from build123d import *

# Parameters (mm, degrees)
SKETCH_1_W          = 49
SKETCH_1_H          = 63
EXTRUDE_1_DEPTH     = 4
SKETCH_2_W          = 45
SKETCH_2_H          = 4
SKETCH_2_W_2        = 4
SKETCH_2_H_2        = 59
EXTRUDE_2_DEPTH     = 26
SKETCH_3_W          = 14
SKETCH_3_H          = 8
SKETCH_3_W_2        = 30
EXTRUDE_3_DEPTH     = 7.2
SKETCH_5_R          = 5.3
CUT_EXTRUDE_1_DEPTH = 4
SKETCH_7_W          = 1.7
SKETCH_7_H          = 1.7
CUT_EXTRUDE_3_DEPTH = 6
SKETCH_8_W          = 1.7
SKETCH_8_H          = 1.7
CUT_EXTRUDE_4_DEPTH = 6
SKETCH_9_W          = 1.7
SKETCH_9_H          = 1.7
CUT_EXTRUDE_5_DEPTH = 6
FILLET_1_R          = 1
SKETCH_6_W          = 1.7
SKETCH_6_H          = 1.7
CUT_EXTRUDE_7_DEPTH = 5
SKETCH_10_W         = 15
SKETCH_10_H         = 27.7
EXTRUDE_4_DEPTH     = 2
CUT_EXTRUDE_8_DEPTH = 13
SKETCH_12_W         = 1.7
SKETCH_12_H         = 1.7
CUT_EXTRUDE_9_DEPTH = 5


with BuildPart() as part:
    # Эскиз1 → Бобышка-Вытянуть1 (new body)
    with BuildSketch(Plane.XY):
        with Locations((2.204545455, -4.295454545)):
            Rectangle(SKETCH_1_W, SKETCH_1_H)
    extrude(amount=EXTRUDE_1_DEPTH)

    # Эскиз2 → Бобышка-Вытянуть2 (add)
    with BuildSketch(Plane(origin=(0, 0, 0), x_dir=(-1, 0, 0), z_dir=(0, 0, -1))):
        with Locations((-0.204545455, 25.204545455)):
            Rectangle(SKETCH_2_W, SKETCH_2_H)
        with Locations((-24.704545455, -6.295454545)):
            Rectangle(SKETCH_2_W_2, SKETCH_2_H_2)
        with Locations((-24.704545455, 25.204545455)):
            Rectangle(SKETCH_2_W_2, SKETCH_2_H)
    extrude(amount=EXTRUDE_2_DEPTH)

    # Эскиз3 → Бобышка-Вытянуть3 (add)
    with BuildSketch(Plane(origin=(0, 0, 0), x_dir=(-1, 0, 0), z_dir=(0, 0, -1))):
        with Locations((-15.704545455, 19.204545455)):
            Rectangle(SKETCH_3_W, SKETCH_3_H)
        with Locations((-7.704545455, -23.795454545)):
            Rectangle(SKETCH_3_W_2, SKETCH_3_H)
    extrude(amount=EXTRUDE_3_DEPTH)

    # Эскиз5 → Вырез-Вытянуть1 (cut)
    with BuildSketch(Plane.ZY.offset(-22.704545455)):
        with Locations((-13, 9.204545455)):
            Circle(SKETCH_5_R)
    extrude(amount=-CUT_EXTRUDE_1_DEPTH, mode=Mode.SUBTRACT)

    # Эскиз7 → Вырез-Вытянуть3 (cut)
    with BuildSketch(Plane.ZY.offset(22.295454545)):
        with Locations((1.75, 24.954545455)):
            Rectangle(SKETCH_7_W, SKETCH_7_H)
    extrude(amount=-CUT_EXTRUDE_3_DEPTH, mode=Mode.SUBTRACT)

    # Эскиз8 → Вырез-Вытянуть4 (cut)
    with BuildSketch(Plane.XZ.offset(35.795454545)):
        with Locations((24.454545455, 1.75)):
            Rectangle(SKETCH_8_W, SKETCH_8_H)
    extrude(amount=-CUT_EXTRUDE_4_DEPTH, mode=Mode.SUBTRACT)

    # Эскиз9 → Вырез-Вытянуть5 (cut)
    with BuildSketch(Plane(origin=(0, 0, -26), x_dir=(-1, 0, 0), z_dir=(0, 0, -1))):
        with Locations((-24.454545455, 24.954545455)):
            Rectangle(SKETCH_9_W, SKETCH_9_H)
    extrude(amount=-CUT_EXTRUDE_5_DEPTH, mode=Mode.SUBTRACT)

    # Скругление1
    fillet_1_edges = [part.edges().sort_by_distance(p)[0] for p in [
        (26.704545455, -4.295454545, 4),
        (2.204545455, 27.204545455, 4),
        (26.704545455, 27.204545455, -11),
    ]]
    fillet(fillet_1_edges, radius=FILLET_1_R)

    # Эскиз6 → Вырез-Вытянуть7 (cut)
    with BuildSketch(Plane(origin=(26.704545455, 0, 0), x_dir=(0, 0, -1), z_dir=(1, 0, 0))):
        with Locations((13, -4.945454545)):
            Rectangle(SKETCH_6_W, SKETCH_6_H)
        with Locations((13, -26.945454545)):
            Rectangle(SKETCH_6_W, SKETCH_6_H)
    extrude(amount=-CUT_EXTRUDE_7_DEPTH, mode=Mode.SUBTRACT)

    # Эскиз10 → Бобышка-Вытянуть4 (add)
    with BuildSketch(Plane.ZY.offset(-22.704545455)):
        with Locations((-7.5, -15.945454545)):
            Rectangle(SKETCH_10_W, SKETCH_10_H)
    extrude(amount=EXTRUDE_4_DEPTH)

    # Эскиз11 → Вырез-Вытянуть8 (cut)
    with BuildSketch(Plane(origin=(0, 27.204545455, 0), x_dir=(1, 0, 0), z_dir=(0, 1, 0))):
        with BuildLine():
            Line((2.704545455, 4), (1.704545455, 4))
            ThreePointArc((1.704545455, 4), (0.997438673, 4.292893219), (0.704545455, 5))
            Line((0.704545455, 5), (0.704545455, 21))
            ThreePointArc((0.704545455, 21), (0.997438673, 21.707106781), (1.704545455, 22))
            Line((1.704545455, 22), (2.704545455, 22))
            ThreePointArc((2.704545455, 22), (3.411652236, 21.707106781), (3.704545455, 21))
            Line((3.704545455, 21), (3.704545455, 5))
            ThreePointArc((3.704545455, 5), (3.411652236, 4.292893219), (2.704545455, 4))
        make_face()
        with BuildLine():
            Line((-3.295454545, 4), (-4.295454545, 4))
            ThreePointArc((-4.295454545, 4), (-5.002561327, 4.292893219), (-5.295454545, 5))
            Line((-5.295454545, 5), (-5.295454545, 21))
            ThreePointArc((-5.295454545, 21), (-5.002561327, 21.707106781), (-4.295454545, 22))
            Line((-4.295454545, 22), (-3.295454545, 22))
            ThreePointArc((-3.295454545, 22), (-2.588347764, 21.707106781), (-2.295454545, 21))
            Line((-2.295454545, 21), (-2.295454545, 5))
            ThreePointArc((-2.295454545, 5), (-2.588347764, 4.292893219), (-3.295454545, 4))
        make_face()
        with BuildLine():
            Line((-9.295454545, 4), (-10.295454545, 4))
            ThreePointArc((-10.295454545, 4), (-11.002561327, 4.292893219), (-11.295454545, 5))
            Line((-11.295454545, 5), (-11.295454545, 21))
            ThreePointArc((-11.295454545, 21), (-11.002561327, 21.707106781), (-10.295454545, 22))
            Line((-10.295454545, 22), (-9.295454545, 22))
            ThreePointArc((-9.295454545, 22), (-8.588347764, 21.707106781), (-8.295454545, 21))
            Line((-8.295454545, 21), (-8.295454545, 5))
            ThreePointArc((-8.295454545, 5), (-8.588347764, 4.292893219), (-9.295454545, 4))
        make_face()
        with BuildLine():
            Line((-15.295454545, 4), (-16.295454545, 4))
            ThreePointArc((-16.295454545, 4), (-17.002561327, 4.292893219), (-17.295454545, 5))
            Line((-17.295454545, 5), (-17.295454545, 21))
            ThreePointArc((-17.295454545, 21), (-17.002561327, 21.707106781), (-16.295454545, 22))
            Line((-16.295454545, 22), (-15.295454545, 22))
            ThreePointArc((-15.295454545, 22), (-14.588347764, 21.707106781), (-14.295454545, 21))
            Line((-14.295454545, 21), (-14.295454545, 5))
            ThreePointArc((-14.295454545, 5), (-14.588347764, 4.292893219), (-15.295454545, 4))
        make_face()
    extrude(amount=-CUT_EXTRUDE_8_DEPTH, mode=Mode.SUBTRACT)

    # Эскиз12 → Вырез-Вытянуть9 (cut)
    with BuildSketch(Plane(origin=(0, 0, -7.2), x_dir=(-1, 0, 0), z_dir=(0, 0, -1))):
        with Locations((-13.654545455, 21.254545455)):
            Rectangle(SKETCH_12_W, SKETCH_12_H)
        with Locations((-13.654545455, -24.095454545)):
            Rectangle(SKETCH_12_W, SKETCH_12_H)
    extrude(amount=-CUT_EXTRUDE_9_DEPTH, mode=Mode.SUBTRACT)


solid = part.part
Can you work these out from the model? Positions are in its coordinate system, mm. A direction names the side the tool comes from. Give positions to 0.01 mm unless a question says otherwise; leave off trailing zeros. Write each loop counter-clockwise with the first axis right and the second up, starting at its lowest first coordinate (ties: lowest second). Pieces come first, ordered by that corner, then holes. Notation, with made-up numbers: (68.5, 29) -> (93.5, 29) arc R36 cw to (93.5, 63) -> close; hole circle Ø6 at (43.25, 30). An arc over 180 degrees is marked (long way). Answer as a JSON object with one key per item and string values. Group by question number.
Item 1: Suppose I cut it at C-C (z = -13). State how many separate pieces and enclosed holes the cut face has, plus the area to 3 significant figures.
Item 2: Please list where these lines run through material, in increasing order: line 1 (Y direction, x = 24.2, z = -13); line 2 (Z direction, x = 3.5, y = -19.5); line 3 (X direction, y = -3.5, z = -3.5). Write a range as [from, to].
Item 3: We'd pull the mould along Y, two halves only. Please class faces 1 (the face through (25, -27, -12.15)), 2 (the face through (22, -29.795, -8)), 3 (the face through (-14.295, 25, -13)), 4 (the face through (7, 27.205, -11)): +Y half, -Y half, draft (parallel to the pull), parting line (faces both ways), or undercut.
Item 4: Suppose I cut it at B-B (x = -12). Please give me the cut outline in (y, z), plus the area to 3 significant figures.
Item 5: For faces 5 (the face through (22.705, -27, -13)), 6 (the face through (-8.295, 25, -13)), 7 (the face through (24, -33, 2.6)), which set-ups out of +Z, -Z, +X, -X, +Y, -Y let a thin tool reach every point of the face, with its end or its side?
Item 6: I'm going to push flat-ended pins straight in: P1, Ø0.8, axis at x = 14, y = 21.5, coming from the -Z side; P2, Ø12, axis at x = -1.5, y = -10, coming from the -Z side; P3, Ø1.5, axis at x = 5.5, y = -25, coming from the -Z side. Where does each tip first touch, or does it pass through?
Item 7: Suppose I cut it at D-D (y = 18). Please give me the cut outline in (x, z), plus the area to 3 significant figures.
Item 8: Suppose I cut it at A-A (y = -0.5). Please give me the cut outline in (x, z).
Findings:
{
 "1": {"separate pieces": "6", "enclosed holes": "0", "area": "383 mm²"},
 "2": {"line 1": "y = [-35.8, -27.8], [-26.1, -5.8], [-4.1, 3.9], [14.5, 27.2]", "line 2": "z = [0, 4]", "line 3": "x = [20.7, 26.7]"},
 "3": {"face 1": "undercut", "face 2": "-Y half", "face 3": "draft", "face 4": "+Y half"},
 "4": {"outline": "(-35.8, 0) -> (23.2, 0) -> (23.2, -26) -> (27.2, -26) -> (27.2, 3) arc R1 ccw to (26.2, 4) -> (-35.8, 4) -> close", "area": "356 mm²"},
 "5": {"face 5": "+X", "face 6": "+Y, -Y", "face 7": "-Y"},
 "6": {"P1": "stops at z = -2.2", "P2": "stops at z = 0", "P3": "stops at z = -7.2"},
 "7": {"outline": "(-22.3, 0) -> (8.7, 0) -> (8.7, -7.2) -> (22.7, -7.2) -> (22.7, -26) -> (26.7, -26) -> (26.7, 3) arc R1 ccw to (25.7, 4) -> (-22.3, 4) -> close", "area": "401 mm²"},
 "8": {"outline": "(-22.3, 0) -> (22.7, 0) -> (22.7, -26) -> (26.7, -26) -> (26.7, 3) arc R1 ccw to (25.7, 4) -> (-22.3, 4) -> close"}
}
